Check sheet for the drawn part. Datum: minimum x, y, z corner. Units: mm. A direction names the side the tool comes from. Round coordinates to 2 decimals unless told otherwise and drop trailing zeros. Loops run counter-clockwise (first coordinate to the right, second up) from the corner with the lowest first, then second, coordinate; pieces in that order, holes last.
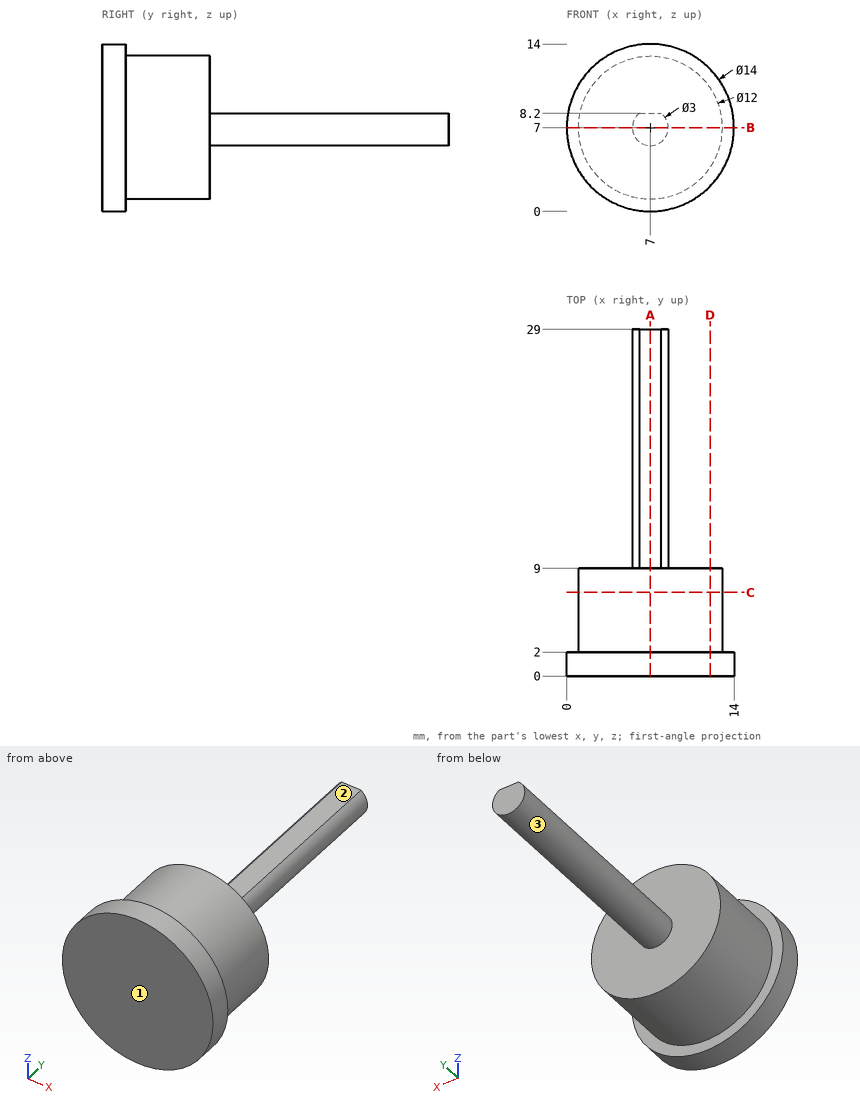
1) Sectioned sample at C-C, the plane y = 7. Record the cut outline in (x, z), then the cut area to 3 significant figures.
Report:
outline: circle Ø12 at (7, 7)
area: 113 mm2
2) Sectioned sample at D-D, the plane x = 12. Record the cut outline in (y, z), then the cut area to 3 significant figures.
Report:
outline: (0, 2.1) - (2, 2.1) - (2, 3.68) - (9, 3.68) - (9, 10.32) - (2, 10.32) - (2, 11.9) - (0, 11.9) - close
area: 66.0 mm2
3) Gauge pin test, flat ends, axial feed: pin 1 (4 mm diameter, centred on y = 9.5, z = 10, fed in from +X) (3 decimals); pin 2 (0.5 mm diameter, centred on x = 6.5, y = 15, fed in from +Z); pin 3 (3 mm diameter, centred on y = 15, z = 3.5, fed in from -X); pin 4 (2 mm diameter, centred on y = 19, z = 7.5, fed in from +X). Record the tip position at first contact, or that the pin passes through.
Report:
pin 1: stops at x = 12.905
pin 2: stops at z = 8.2
pin 3: passes through
pin 4: stops at x = 8.5
4) Access from +Z, -Z, +X, -X, +Y, -Y to the whole of each face (thin tool, end or side, straight path). Record for the marked faces 1, 2 and 3.
Report:
face 1: +Z, -Z, +X, -X, -Y
face 2: +Z, +X, -X, +Y
face 3: +Y
5) Sectioned sample at B-B, the plane z = 7. Record the cut outline in (x, y), then the cut area to 3 significant figures.
Report:
outline: (0, 0) - (14, 0) - (14, 2) - (13, 2) - (13, 9) - (8.5, 9) - (8.5, 29) - (5.5, 29) - (5.5, 9) - (1, 9) - (1, 2) - (0, 2) - close
area: 172 mm2
6) Scan lines: line 1 along Y through (x, z) = (4.75, 6.25); line 2 along Y through (x, z) = (2.25, 2.25); line 3 along Z through (x, y) = (7.75, 11.75). Record each from-to range of solid material in increasing order.
Report:
line 1: y = 0 to 9
line 2: y = 0 to 2
line 3: z = 5.7 to 8.2
7) Sectioned sample at A-A, the plane x = 7. Record the cut outline in (y, z), then the cut area to 3 significant figures.
Report:
outline: (0, 0) - (2, 0) - (2, 1) - (9, 1) - (9, 5.5) - (29, 5.5) - (29, 8.2) - (9, 8.2) - (9, 13) - (2, 13) - (2, 14) - (0, 14) - close
area: 166 mm2
